from build123d import *

# Parameters (mm, degrees)
SKETCH1_R           = 9.5
SKETCH1_R_2         = 6
SKETCH1_R_3         = 1.25
BOSS_EXTRUDE1_DEPTH = 2
BOSS_EXTRUDE2_START = 2
SKETCH1_3_R         = 6
BOSS_EXTRUDE2_DEPTH = 1
BOSS_EXTRUDE2_TAPER = 45
SKETCH2_R           = 8.5
CUT_EXTRUDE1_DEPTH  = 0.25
CUT_EXTRUDE1_DRAFT  = -84
SKETCH1_4_R         = 1.25
CUT_EXTRUDE2_DEPTH  = 40.25
FILLET1_R           = 0.5


with BuildPart() as part:
    # Sketch1 → Boss-Extrude1 (new body)
    # profile 1 of 2: a face of its own
    with BuildSketch(Plane.XY):
        Circle(SKETCH1_R)
        Circle(SKETCH1_R_2, mode=Mode.SUBTRACT)
    # profile 2 of 2: a face of its own
    with BuildSketch(Plane.XY):
        Circle(SKETCH1_R_2)
        Circle(SKETCH1_R_3, mode=Mode.SUBTRACT)
    extrude(amount=BOSS_EXTRUDE1_DEPTH)

    # Sketch1<3> → Boss-Extrude2 (add)
    with BuildSketch(Plane.XY.offset(BOSS_EXTRUDE2_START)):
        Circle(SKETCH1_3_R)
    extrude(amount=BOSS_EXTRUDE2_DEPTH, taper=BOSS_EXTRUDE2_TAPER)


with BuildPart() as cut_extrude1_tool:
    # Sketch2 → Cut-Extrude1 (with draft: the straight prism first)
    with BuildSketch(Plane(origin=(0, 0, 0), x_dir=(-1, 0, 0), z_dir=(0, 0, -1))):
        Circle(SKETCH2_R)
    extrude(amount=-CUT_EXTRUDE1_DEPTH)
    # Cut-Extrude1: the draft: its side faces are tilted about the plane it starts from
    cut_extrude1_sides = [cut_extrude1_tool.faces().sort_by_distance(p)[0] for p in [
        (8.5, 0, 0.125),
    ]]
    draft(cut_extrude1_sides, Plane(origin=(0, 0, 0), x_dir=(-1, 0, 0), z_dir=(0, 0, -1)), CUT_EXTRUDE1_DRAFT)


with BuildPart() as part_1:
    add(part.part)

    # Cut-Extrude1: cut by cut_extrude1_tool
    add(cut_extrude1_tool.part, mode=Mode.SUBTRACT)

    # Sketch1<4> → Cut-Extrude2 (cut)
    with BuildSketch(Plane.XY):
        with Locations(Location((0, 0, 0), (0, 0, 180))):
            Circle(SKETCH1_4_R)
    extrude(amount=CUT_EXTRUDE2_DEPTH, mode=Mode.SUBTRACT)

    # Fillet1
    fillet1_edges = [part_1.edges().sort_by_distance(p)[0] for p in [
        (-9.5, 0, 0),
        (-9.5, 0, 2),
    ]]
    fillet(fillet1_edges, radius=FILLET1_R)


solid = part_1.part
Build history of the part. All positions in model axes, mm. A direction names the side the tool comes from. Round coordinates to 2 decimals unless told otherwise and drop trailing zeros. Write each loop counter-clockwise with the first axis right and the second up, starting at its lowest first coordinate (ties: lowest second). Pieces come first, ordered by that corner, then holes. Notation, with made-up numbers: M 86,32.5 L 139,32.5 A12 ccw 139,44.5 Z; hole C 76.25,-19 d4. An arc over 180 degrees is marked long. Answer in a Markdown table with one row per item.
1. Saw through at C-C (z = 2.3). List the corners of the cut face in (x, y).
Geometry check:
| item | result |
|---|---|
| outline | C 0,0 d11.4; hole C 0,0 d2.5 |
2. Mould opens along X. For faces 1 (the face through (1, -1, 3)), 2 (the face through (0.1, 1.4, 0.25)), 3 (the face through (4.38, -8.43, 0.99)) say: +X half, -X half, draft (parallel to the pull), parting line (faces both ways), or undercut.
Geometry check:
| item | result |
|---|---|
| face 1 | draft |
| face 2 | undercut |
| face 3 | parting line |
3. Which spindle directions (+Z, -Z, +X, -X, +Y, -Y) get a long thin tool onto all of the face, cutting with end or side? Do faces 4 (the face through (0.082, 1.247, 1.606)), 5 (the face through (2, -6, 2)). Say none if no direction does.
Geometry check:
| item | result |
|---|---|
| face 4 | +Z, -Z |
| face 5 | +Z |
4. Flat gauge pins, fed straight in: P1, Ø1, axis at x = -5.5, y = 2, coming from the -Z side; P2, Ø1.5, axis at x = -5.5, y = 3.5, coming from the -Z side. Where does each tip first touch, or does it go through?
Geometry check:
| item | result |
|---|---|
| P1 | z = 0.23 |
| P2 | z = 0.13 |
5. Saw through at A-A (y = 0). List the corners of the cut face in (x, z), and give its area (3 significant figures).
Geometry check:
| item | result |
|---|---|
| outline | M -9.5,0.5 A0.5 ccw -9,0 L -8.5,0 L -6.12,0.25 L -1.25,0.25 L -1.25,3 L -5,3 L -6,2 L -9,2 A0.5 ccw -9.5,1.5 Z; M 1.25,0.25 L 6.12,0.25 L 8.5,0 L 9,0 A0.5 ccw 9.5,0.5 L 9.5,1.5 A0.5 ccw 9,2 L 6,2 L 5,3 L 1.25,3 Z |
| area | 38.3 mm2 |
6. Probe L1, parallel to Z at x = -1, y = -1.5; L2, parallel to Z at x = -8, y = -3.25; L3, parallel to Y at x = 0, z = 2.3. List the from-to ranges inside material, lowest first. Write a range as [from, to].
Geometry check:
| item | result |
|---|---|
| L1 | [0.25, 3] |
| L2 | [0, 2] |
| L3 | [-5.7, -1.25], [1.25, 5.7] |
